Could you check a few things on this model? Use its own coordinates, in mm. Give positions to 0.01 mm unless a question says otherwise; leave off trailing zeros. Order: outer loops, then holes, each group sorted by start corner. A loop starts at its lowest first (then second) coordinate and runs counter-clockwise, first axis right, second up. Notation, with made-up numbers: (1, 78) -> (45, 78) arc R24 cw to (45, 99) -> close; hole circle Ø3 at (79, -11). An arc over 180 degrees is marked (long way). One line per item, written item: value.
```python
from build123d import *

# Parameters (mm, degrees)
F0_R     = 11.919915
F1_DEPTH = 21
F3_DEPTH = 2
F5_DEPTH = 25


with BuildPart() as f1:
    # F0 (on Top) → F1 (new body)
    with BuildSketch(Plane.XY):
        with Locations((-8.941904, 13.841942)):
            Circle(F0_R)
    extrude(amount=F1_DEPTH)

    # F2 (on face) → F3 (join)
    with BuildSketch(Plane.XY.offset(21)):
        with BuildLine():
            ThreePointArc((-8.255348, 1.941816), (-0.273915, 5.659623), (2.978011, 13.841942))
            ThreePointArc((2.978011, 13.841942), (-0.273915, 22.024261), (-8.255348, 25.742068))
            ThreePointArc((-8.255348, 25.742068), (-20.861818, 13.841942), (-8.255348, 1.941816))
        make_face()
        with BuildLine():
            ThreePointArc((-8.255348, 25.742068), (-0.273915, 22.024261), (2.978011, 13.841942))
            Line((2.978011, 13.841942), (63.745973, 13.841942))
            ThreePointArc((63.745973, 13.841942), (66.038754, 19.159212), (71.479256, 21.141927))
            Line((71.479256, 21.141927), (-8.255348, 25.742068))
        make_face()
        with BuildLine():
            Line((63.745973, 13.841942), (2.978011, 13.841942))
            ThreePointArc((2.978011, 13.841942), (-0.273915, 5.659623), (-8.255348, 1.941816))
            Line((-8.255348, 1.941816), (71.479256, 6.541957))
            ThreePointArc((71.479256, 6.541957), (66.038754, 8.524672), (63.745973, 13.841942))
        make_face()
        with BuildLine():
            ThreePointArc((71.479256, 21.141927), (66.038754, 19.159212), (63.745973, 13.841942))
            ThreePointArc((63.745973, 13.841942), (66.038754, 8.524672), (71.479256, 6.541957))
            ThreePointArc((71.479256, 6.541957), (76.375366, 8.8226), (78.37022, 13.841942))
            ThreePointArc((78.37022, 13.841942), (76.375366, 18.861284), (71.479256, 21.141927))
        make_face()
    extrude(amount=F3_DEPTH)

    # F4 (on face) → F5 (cut)
    with BuildSketch(Plane.XY.offset(23)):
        with BuildLine():
            Line((28.891168, 8.841942), (71.058096, 8.841942))
            ThreePointArc((71.058096, 8.841942), (76.052672, 14.074788), (70.59291, 18.820255))
            Line((70.59291, 18.820255), (28.893769, 18.841941))
            ThreePointArc((28.893769, 18.841941), (23.891169, 13.843242), (28.891168, 8.841942))
        make_face()
    extrude(amount=-F5_DEPTH, mode=Mode.SUBTRACT)


solid = f1.part
```
1) Suppose I cut it at B-B, the plane x = 48.5. Write out the boundary of the cut face in (y, z).
Answer below:
outline: (5.22, 21) -> (8.84, 21) -> (8.84, 23) -> (5.22, 23) -> close; (18.83, 21) -> (22.47, 21) -> (22.47, 23) -> (18.83, 23) -> close
2) Suppose I cut it at C-C, the plane y = 22.25. Write out the boundary of the cut face in (x, z).
Answer below:
outline: (-17.39, 0) -> (-0.49, 0) -> (-0.49, 21) -> (52.27, 21) -> (52.27, 23) -> (-17.39, 23) -> close
3) We'd pull the mould along Y, two halves only. Please class faces 1 (the flat face through (50, 8.842, 22)), 2 (the flat face through (31.05, 4.21, 21.99)), 3 (the flat face through (-9, 14, 0)), 4 (the cylindrical face through (23.892, 13.953, 22.014)): +Y half, -Y half, draft (parallel to the pull), parting line (faces both ways), or undercut.
Answer below:
face 1: undercut
face 2: -Y half
face 3: draft
face 4: undercut
4) Suppose I cut it at D-D, the plane x = 63.5. Write out the boundary of the cut face in (y, z).
Answer below:
outline: (6.08, 21) -> (8.84, 21) -> (8.84, 23) -> (6.08, 23) -> close; (18.82, 21) -> (21.6, 21) -> (21.6, 23) -> (18.82, 23) -> close
5) If I drill on line 1 along Z through (x, y) = (20, 21); line 2 along X through (y, z) = (10.25, 20.75); line 3 along Y through (x, z) = (0.5, 14), over which ranges is the centre line in solid material (lowest first)?
Answer below:
line 1: z = 21 to 23
line 2: x = -20.31 to 2.42
line 3: y = 6.57 to 21.12
6) For P1, Ø1.6, axis at x = 57.5, z = 22.5, coming from the +Y side; P2, Ø8, axis at x = -2.5, z = 14.5, coming from the -Y side; P3, Ø4, axis at y = 23, z = 16.5, coming from the +X side; P4, Ø8, axis at x = 9.5, z = 11, coming from the -Y side, each with a flat end and sliding along its axis, tell me the tip position at first contact or that it passes through.
Answer below:
P1: stops at y = 21.99
P2: stops at y = 2.17
P3: stops at x = 0.59
P4: passes through
7) Suppose I cut it at A-A, the plane y = 16. Write out the boundary of the cut face in (x, z), then the cut area to 3 significant figures.
Answer below:
outline: (-20.66, 0) -> (2.78, 0) -> (2.78, 21) -> (24.38, 21) -> (24.38, 23) -> (-20.66, 23) -> close; (75.57, 21) -> (78.04, 21) -> (78.04, 23) -> (75.57, 23) -> close
area: 587 mm2
